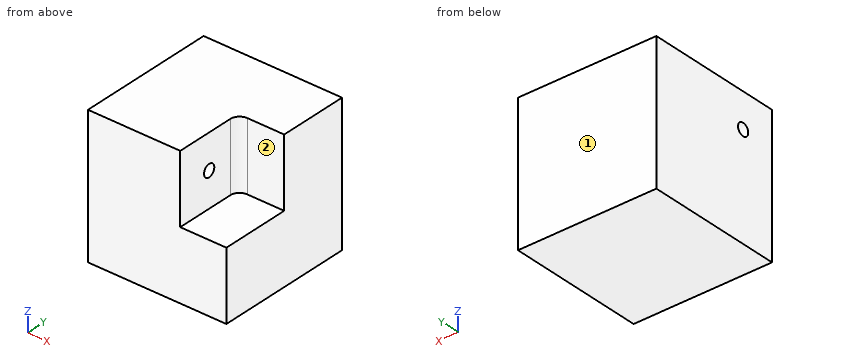
```python
from build123d import *

# Parameters (mm, degrees)
F0_W     = 76.2
F0_H     = 76.2
F1_DEPTH = 38.1
F2_W     = 25.4
F2_H     = 38.1
F3_DEPTH = 38.1
F5_D     = 6.7564
F6_R     = 5.08


with BuildPart() as f1:
    # F0 (on Front) → F1 (new body, symmetric)
    with BuildSketch(Plane.XZ):
        Rectangle(F0_W, F0_H)
    extrude(amount=F1_DEPTH, both=True)

    # F2 (on face) → F3 (cut)
    with BuildSketch(Plane.XZ.offset(38.1)):
        with Locations((25.4, 19.05)):
            Rectangle(F2_W, F2_H)
    extrude(amount=-F3_DEPTH, mode=Mode.SUBTRACT)

    # F5 (through all)
    with Locations(Plane.YZ.offset(12.7)):
        with Locations((-19.05, 19.05)):
            Hole(F5_D / 2)

    # F6
    f6_edges = [f1.edges().sort_by_distance(p)[0] for p in [
        (12.7, 0, 19.05),
    ]]
    fillet(f6_edges, radius=F6_R)


solid = f1.part
```
Can you work these out from the model? Positions are in its coordinate system, mm. Face numbers are marked on the shaded views. A direction names the side the tool comes from. Round coordinates to 2 decimals unless told otherwise and drop trailing zeros. Loops run counter-clockwise (first coordinate to the right, second up) from the corner with the lowest first, then second, coordinate; pieces in that order, holes last. Notation, with made-up numbers: M -14,-6 L 23,-6 A25 cw 23,31 Z; hole C 67.5,53 d1. An arc over 180 degrees is marked long. Write item = value, one per line. Start each with the question number.
(1) Suppose I cut it at A-A on z = 19.05. Write out the boundary of the cut face in (x, y).
(2) Which directions (+Z, -Z, +X, -X, +Y, -Y) give clear straight access to the entire face, cutting with the end or side of a thin tool? Please do the marked faces 1 and 2.
(3) Suppose I cut it at B-B on y = -19.05. Write out the boundary of the cut face in (x, z), plus the area to 3 significant figures.
(4) I need wall thicknesses on line 1 along Z through (x, y) = (-8, -19); line 2 along Z through (x, y) = (17, -7); line 3 along X through (y, z) = (-25.5, 9.5). Which ranges of each line are inside material? Lowest first, please.
(5) I'm going to push flat-ended pins straight in: P1, Ø8, axis at y = -19.05, z = 19.05, coming from the +X side; P2, Ø7.5, axis at x = 30.5, y = -25, coming from the +Z side; P3, Ø22.5, axis at x = 27.5, z = 27.5, coming from the -Y side. Where does each tip first touch, or does it pass through?
(6) Suppose I cut it at C-C on z = 32. Write out the boundary of the cut face in (x, y).
Answer block:
q1.outline = M -38.1,-38.1 L 12.7,-38.1 L 12.7,-22.43 L -38.1,-22.43 Z; M -38.1,-15.67 L 12.7,-15.67 L 12.7,-5.08 A5.08 cw 17.78,0 L 38.1,0 L 38.1,38.1 L -38.1,38.1 Z
q2.face_1 = +Z, -Z, +X, -X, +Y
q2.face_2 = +Z, +X, -Y
q3.outline = M -38.1,-38.1 L 38.1,-38.1 L 38.1,0 L 12.7,0 L 12.7,15.67 L -38.1,15.67 Z; M -38.1,22.43 L 12.7,22.43 L 12.7,38.1 L -38.1,38.1 Z
q3.area = 4,500 mm²
q4.line_1 = -38.1 to 15.67, 22.43 to 38.1
q4.line_2 = -38.1 to 0
q4.line_3 = -38.1 to 12.7
q5.P1 = 12.7
q5.P2 = 0
q5.P3 = -0.24
q6.outline = M -38.1,-38.1 L 12.7,-38.1 L 12.7,-5.08 A5.08 cw 17.78,0 L 38.1,0 L 38.1,38.1 L -38.1,38.1 Z
